Part print with two shaded views. Sizes in mm from the minimum x, y, z corner. A direction names the side the tool comes from. Give positions to 0.01 mm unless a question says otherwise; leave off trailing zeros. Order: outer loops, then holes, each group sorted by start corner. A loop starts at its lowest first (then second) coordinate and runs counter-clockwise, first axis right, second up.
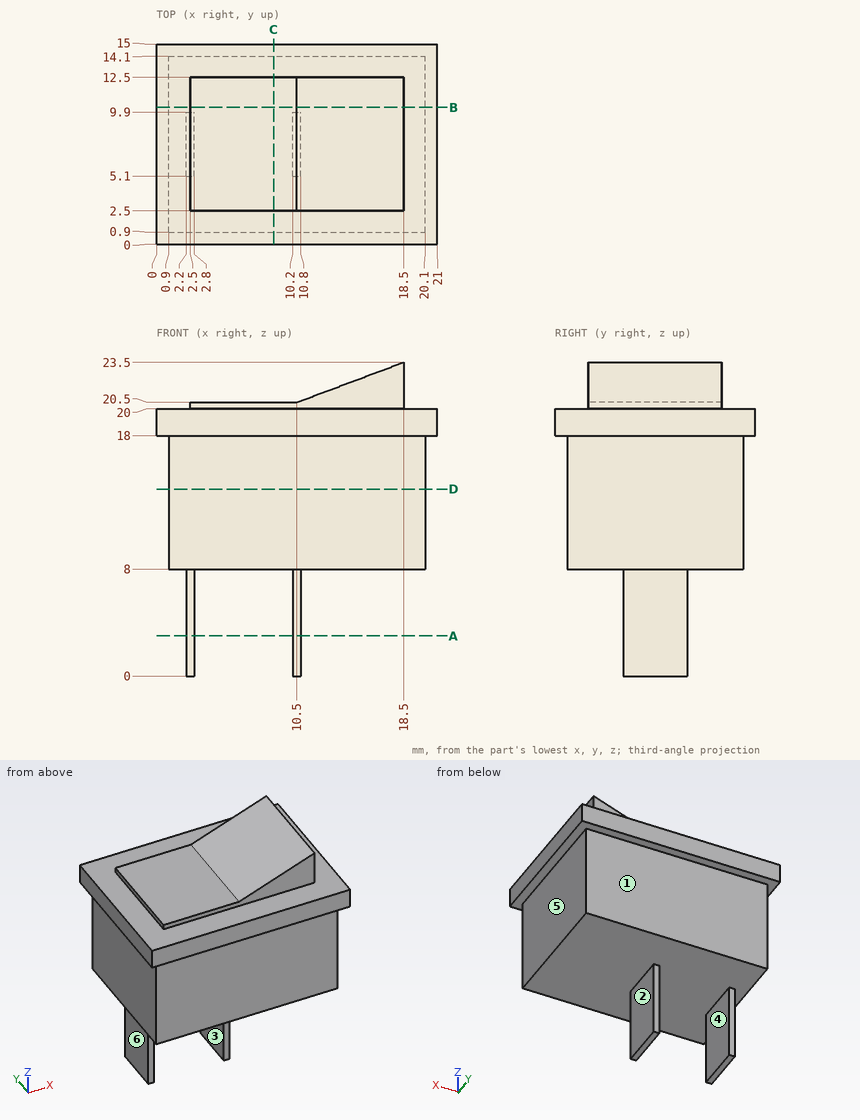
Item 1: Two-plate mould, pull along X, no slides. Class the marked faces 4, 5 and 6: released by +X, released by -X, zero draft, split by the parting line, or undercut.
Item 2: Slice it at C-C (x = 8.75). Give the cut face in (y, z).
Item 3: Wall check: L1, parallel to X at y = 6.5, z = 9; L2, parallel to Y at x = 12.5, z = 17.5; L3, parallel to Z at x = 4, y = 5. Give the ranges that are in metal, low to high.
Item 4: Tool access for the marked faces 1, 2 and 3: list every direction of +Z, -Z, +X, -X, +Y, -Y with a clear straight run to the whole face (end or side of a thin tool).
Item 5: Drop flat-ended pins along their axis: pin 1 Ø5 at (x, z) = (8, 13) entering from -Y; pin 2 Ø6 at (x, y) = (12.5, 11.5) entering from +Z (3 decimals); pin 3 Ø5 at (y, z) = (10.5, 13.5) entering from +X; pin 4 Ø6 at (y, z) = (7.5, 15.5) entering from +X. Give the stop position or say it passes through.
Item 6: Slice it at B-B (y = 10.25). Give the cut face in (x, z).
Item 7: Slice it at D-D (z = 14). Give the cut face in (x, y).
Item 8: Slice it at A-A (z = 3). Give the cut face in (x, y).
A:
1. face 4: undercut
1. face 5: released by +X
1. face 6: released by -X
2. outline: (0, 18) - (0.9, 18) - (0.9, 8) - (14.1, 8) - (14.1, 18) - (15, 18) - (15, 20) - (12.5, 20) - (12.5, 20.5) - (2.5, 20.5) - (2.5, 20) - (0, 20) - close
3. L1: x = 0.9 to 20.1
3. L2: y = 0.9 to 14.1
3. L3: z = 8 to 20.5
4. face 1: -Z, +X, -X, +Y
4. face 2: -Z, +X, +Y, -Y
4. face 3: -Z, +Y, -Y
5. pin 1: stops at y = 0.9
5. pin 2: stops at z = 22.375
5. pin 3: stops at x = 20.1
5. pin 4: stops at x = 21
6. outline: (0, 18) - (0.9, 18) - (0.9, 8) - (20.1, 8) - (20.1, 18) - (21, 18) - (21, 20) - (18.5, 20) - (18.5, 23.5) - (10.5, 20.5) - (2.5, 20.5) - (2.5, 20) - (0, 20) - close
7. outline: (0.9, 0.9) - (20.1, 0.9) - (20.1, 14.1) - (0.9, 14.1) - close
8. outline: (2.2, 5.1) - (2.8, 5.1) - (2.8, 9.9) - (2.2, 9.9) - close; (10.2, 5.1) - (10.8, 5.1) - (10.8, 9.9) - (10.2, 9.9) - close
